```python
from build123d import *

# Parameters (mm, degrees)
SKETCH004_R        = 4
SKETCH001_R        = 6
SKETCH002_R        = 6
EXTRUDE002_DEPTH   = 3
SKETCH005_R        = 3.5
POCKET_DEPTH       = 5
POCKET001_DEPTH    = 1.2
POLARPATTERN_COUNT = 6
FILLET_R           = 1.5


with BuildPart() as revolution:
    # Sketch006 → Revolution (revolve)
    with BuildSketch(Plane.XZ):
        with BuildLine():
            Line((0, 0), (8, 0))
            ThreePointArc((8, 0), (10, 2), (8, 4))
            Line((8, 4), (0, 4))
            Line((0, 4), (0, 0))
        make_face()
    revolve(axis=Axis((0, 0, 0), (0, 0, 1)))


with BuildPart() as loft_body:
    # Sketch004 → Loft section 0
    with BuildSketch(Plane.XY.offset(18)):
        Circle(SKETCH004_R)
    # Sketch001 → Loft section 1
    with BuildSketch(Plane.XY.offset(4)):
        Circle(SKETCH001_R)
    loft()


with BuildPart() as fillet_body:
    # Sketch002 → Extrude002 (new body)
    with BuildSketch(Plane.XY.offset(17)):
        Circle(SKETCH002_R)
    extrude(amount=EXTRUDE002_DEPTH)

    # Sketch005 → Pocket (cut)
    with BuildSketch(Plane.XY.offset(20)):
        Circle(SKETCH005_R)
    extrude(amount=-POCKET_DEPTH, mode=Mode.SUBTRACT)

    # Sketch → Pocket001 (cut)
    with BuildSketch(Plane.XY.offset(20)):
        with BuildLine():
            ThreePointArc((2.53571, 5.437847), (1.298638, 5.857776), (0, 6))
            Line((0, 0), (0, 6))
            Line((0, 0), (2.53571, 5.437847))
        make_face()
    pocket001 = extrude(amount=-POCKET001_DEPTH, mode=Mode.SUBTRACT)

    # PolarPattern: Pocket001 ×6 about axis
    polarpattern_axis = Axis((0, 0, 20), (0, 0, 1))
    for i in range(1, POLARPATTERN_COUNT):
        add(pocket001.rotate(polarpattern_axis, i * 360 / POLARPATTERN_COUNT), mode=Mode.SUBTRACT)

    # Fusion: union Revolution, Loft body
    add(revolution.part)
    add(loft_body.part)

    # Fillet
    fillet_edges = [fillet_body.edges().sort_by_distance(p)[0] for p in [
        (-4.142857, 0, 17),
    ]]
    fillet(fillet_edges, radius=FILLET_R)


solid = fillet_body.part
```
Verification items for the finished model (mm, model axes). A direction names the side the tool comes from. Coordinates: 2 decimals unless noted, no trailing zeros. Write each loop counter-clockwise with the first axis right and the second up, starting at its lowest first coordinate (ties: lowest second). Pieces come first, ordered by that corner, then holes. Notation, with made-up numbers: M -19.75,52 L 3.25,52 A11 ccw 3.25,64 Z; hole C 57.25,45.5 d3. An arc over 180 degrees is marked long. Answer as a JSON object with one key per item and string values. Group by question number.
(1) Material ranges on line 1 (Y direction, x = 0, z = 18.65); line 2 (Z direction, x = 4.25, y = 6.25); line 3 (Z direction, x = 1.75, y = 0.5), recorded low to high.
(2) Tool access check on faces 4 (the face through (-1, -5, 18.8)), 5 (the face through (2.769, -5.323, 18.479)), 6 (the face through (-4.098, -2.366, 19.408)), 7 (the face through (0, 5, 19)), 8 (the face through (-5, 1, 20)). Record the directions out of +Z, -Z, +X, -X, +Y, -Y that give a thin tool (end or side, any length) a straight path to the whole face; none if there is none.
(3) Cross-section at A-A, the plane z = 11. Record the cut outline in (x, y), and give its area (3 significant figures).
(4) Gauge pin test, flat ends, axial feed: pin 1 (8 mm diameter, centred on x = 7, z = 10, fed in from +Y); pin 2 (3 mm diameter, centred on y = -6.5, z = 12, fed in from -X); pin 3 (0.8 mm diameter, centred on x = -4.5, y = -1, fed in from +Z); pin 4 (1.5 mm diameter, centred on y = -4, z = 8.5, fed in from -X). Record the tip position at first contact, or that the pin passes through.
(5) Cross-section at B-B, the plane z = 13.5. Record the cut outline in (x, y), and give its area (3 significant figures).
(6) Release check for a two-part mould opening along Z. For faces 1 (the face through (-2.714, 3.877, 19.408)), 2 (the face through (4, 1, 18.8)), 3 (the face through (4.8, 1.5, 10.8)) record: +Z half, -Z half, draft (parallel to the pull), parting line (faces both ways), or undercut.
Reply:
{
 "1": {"line 1": "-6 to -3.5, 3.5 to 6", "line 2": "0 to 4", "line 3": "0 to 18"},
 "2": {"face 4": "+Z, -Y", "face 5": "+Z", "face 6": "+Z, -X", "face 7": "+Z, +Y", "face 8": "+Z, +X, -X, +Y, -Y"},
 "3": {"outline": "C 0,0 d10", "area": "78.5 mm²"},
 "4": {"pin 1": "y = 4.26", "pin 2": "through", "pin 3": "z = 18.8", "pin 4": "x = -4.27"},
 "5": {"outline": "C 0,0 d9.29", "area": "67.7 mm²"},
 "6": {"face 1": "draft", "face 2": "+Z half", "face 3": "undercut"}
}
